```python
from build123d import *

# Parameters (mm, degrees)
F1_DEPTH  = 2
F3_DEPTH  = 2
F5_DEPTH  = 3.7
F5_FACE_R = 4.65


with BuildPart() as f1:
    # F0 (on Top) → F1 (new body)
    with BuildSketch(Plane.XY):
        with BuildLine():
            Line((-4.516799, 1.105), (-5.3, 1.105))
            Line((-5.3, 1.105), (-5.3, -1.105))
            Line((-5.3, -1.105), (-4.516799, -1.105))
            ThreePointArc((-4.516799, -1.105), (-4.65, 0), (-4.516799, 1.105))
        make_face()
        with BuildLine():
            ThreePointArc((0, 2.95), (-1.649659, 2.445634), (-2.735229, 1.105))
            ThreePointArc((-2.735229, 1.105), (-2.895809, 0.562839), (-2.95, 0))
            ThreePointArc((-2.95, 0), (-2.895809, -0.562839), (-2.735229, -1.105))
            ThreePointArc((-2.735229, -1.105), (-1.649659, -2.445634), (0, -2.95))
            ThreePointArc((0, -2.95), (1.649659, -2.445634), (2.735229, -1.105))
            ThreePointArc((2.735229, -1.105), (2.895809, -0.562839), (2.95, 0))
            ThreePointArc((2.95, 0), (2.895809, 0.562839), (2.735229, 1.105))
            ThreePointArc((2.735229, 1.105), (1.649659, 2.445634), (0, 2.95))
        make_face()
        with BuildLine():
            Line((5.3, 1.105), (4.516799, 1.105))
            ThreePointArc((4.516799, 1.105), (4.61658, 0.5565), (4.65, 0))
            ThreePointArc((4.65, 0), (4.61658, -0.5565), (4.516799, -1.105))
            Line((4.516799, -1.105), (5.3, -1.105))
            Line((5.3, -1.105), (5.3, 1.105))
        make_face()
        with BuildLine():
            Line((-2.735229, 1.105), (-4.516799, 1.105))
            ThreePointArc((-4.516799, 1.105), (-4.65, 0), (-4.516799, -1.105))
            Line((-4.516799, -1.105), (-2.735229, -1.105))
            ThreePointArc((-2.735229, -1.105), (-2.895809, -0.562839), (-2.95, 0))
            ThreePointArc((-2.95, 0), (-2.895809, 0.562839), (-2.735229, 1.105))
        make_face()
        with BuildLine():
            ThreePointArc((4.65, 0), (4.61658, 0.5565), (4.516799, 1.105))
            Line((4.516799, 1.105), (2.735229, 1.105))
            ThreePointArc((2.735229, 1.105), (2.895809, 0.562839), (2.95, 0))
            ThreePointArc((2.95, 0), (2.895809, -0.562839), (2.735229, -1.105))
            Line((2.735229, -1.105), (4.516799, -1.105))
            ThreePointArc((4.516799, -1.105), (4.61658, -0.5565), (4.65, 0))
        make_face()
    extrude(amount=F1_DEPTH)

    # F2 (on face) → F3 (join)
    with BuildSketch(Plane(origin=(0, 0, 0), x_dir=(1, 0, 0), z_dir=(0, 0, -1))):
        with BuildLine():
            Line((-5.3, 1.105), (-5.3, -1.105))
            ThreePointArc((-5.3, -1.105), (-4.408442, -3.142717), (-2.772819, -4.65))
            Line((-2.772819, -4.65), (0, -4.65))
            Line((0, -4.65), (2.772819, -4.65))
            ThreePointArc((2.772819, -4.65), (4.408442, -3.142717), (5.3, -1.105))
            Line((5.3, -1.105), (5.3, 1.105))
            ThreePointArc((5.3, 1.105), (4.408442, 3.142717), (2.772819, 4.65))
            Line((2.772819, 4.65), (0, 4.65))
            Line((0, 4.65), (-2.772819, 4.65))
            ThreePointArc((-2.772819, 4.65), (-4.408442, 3.142717), (-5.3, 1.105))
        make_face()
    extrude(amount=F3_DEPTH)

    # F4 (on face) → F5 (join)
    with BuildSketch(Plane(origin=(0, 0, -2), x_dir=(1, 0, 0), z_dir=(0, 0, -1))):
        with BuildLine():
            ThreePointArc((0, -4.65), (3.288047, -3.288047), (4.65, 0))
            ThreePointArc((4.65, 0), (3.288047, 3.288047), (0, 4.65))
            ThreePointArc((0, 4.65), (-4.65, 0), (0, -4.65))
        make_face()
    extrude(amount=F5_DEPTH)

    # F5_face (on face) → F7 section 0
    with BuildSketch(Plane(origin=(0, 0, -5.7), x_dir=(1, 0, 0), z_dir=(0, 0, -1)), mode=Mode.PRIVATE) as f7_s0:
        Circle(F5_FACE_R)
    loft([Vertex(0, 0, -9), f7_s0.sketch])


solid = f1.part
```
Check sheet for the modelled part. Datum: model origin and axes. Units: mm. A direction names the side the tool comes from. Round coordinates to 2 decimals unless told otherwise and drop trailing zeros. Write each loop counter-clockwise with the first axis right and the second up, starting at its lowest first coordinate (ties: lowest second). Pieces come first, ordered by that corner, then holes. Notation, with made-up numbers: (55.25, 78) -> (63.25, 78) arc R22 cw to (63.25, 89) -> close; hole circle Ø6 at (42, 74). An arc over 180 degrees is marked (long way). One line per question, with ' | ' between items. Start each with the question number.
1. Depth check by flat-ended pin: pin 1 (1.6 mm diameter, centred on x = -3.5, z = 1.5, fed in from +Y); pin 2 (1 mm diameter, centred on x = -3.5, y = 1, fed in from -Z); pin 3 (2 mm diameter, centred on x = 4, z = 0.5, fed in from +Y). Enter the tip coordinate at first touch or a pass-through.
2. Set-up check for faces 1 (the face through (4, 1.105, 1)), 2 (the face through (4, -1.105, 1)), 3 (the face through (5, 0, -2)), 4 (the face through (-0.1, -3.3, 0)): record each of +Z, -Z, +X, -X, +Y, -Y from which the full face is reachable in a straight line by a thin tool's end or side.
3. Sectioned sample at B-B, the plane z = -6.25. Record the cut outline in (x, y) (3 decimals).
4. Scan lines: line 1 along X through (y, z) = (0.5, -7); line 2 along Z through (x, y) = (4.5, 1.5); line 3 along X through (y, z) = (2.25, -4.5). Record each from-to range of solid material in increasing order. Write a range as from..to.
5. Sectioned sample at A-A, the plane z = -4.75. Record the cut outline in (x, y).
Taken from the geometry:
1) pin 1: stops at y = 1.19 | pin 2: stops at z = -6.77 | pin 3: stops at y = 4.41
2) face 1: +Z, +X, +Y | face 2: +Z, +X, -Y | face 3: -Z, +X | face 4: +Z, -Y
3) outline: circle Ø7.75 at (0, 0)
4) line 1: x = -2.77..2.77 | line 2: z = -2..0 | line 3: x = -4.07..4.07
5) outline: (0, -4.65) arc R4.65 ccw to (4.65, 0) arc R4.65 ccw to (0, 4.65) arc R4.65 ccw to start
